Autodesk Inventor part; units mm, degrees
ref_plane "YZ Plane" through (0, 0, 0) normal (1, 0, 0) x (0, 1, 0)
ref_plane "XZ Plane" through (0, 0, 0) normal (0, 1, 0) x (-1, 0, 0)
ref_plane "XY Plane" through (0, 0, 0) normal (0, 0, 1) x (1, 0, 0)
sketch "Sketch1" plane through (0, 0, 0) normal (0, 0, 1) x (1, 0, 0)
  line L0 (14, -20) -> (-14, -20) construction
  line L1 (-14, -20) -> (-14, 20) construction
  line L2 (-14, 20) -> (14, 20) construction
  line L3 (14, 20) -> (14, -20) construction
  line L4 (14, -20) -> (-14, 20) construction
  line L5 (-14, -20) -> (14, 20) construction
  circle A0 centre (-14, 20) radius 2.25
  circle A1 centre (14, 20) radius 2.25
  circle A2 centre (14, -20) radius 2.25
  circle A3 centre (-14, -20) radius 2.25
  line L6 (0, 0) -> (0, -8.85) construction
  circle A4 centre (0, -8.85) radius 10
  line L7 (20.06, -29.05) -> (-20.06, -29.05)
  line L8 (-20.06, -29.05) -> (-20.06, 29.05)
  line L9 (-20.06, 29.05) -> (20.06, 29.05)
  line L10 (20.06, 29.05) -> (20.06, -29.05)
  line L11 (20.06, -29.05) -> (-20.06, 29.05) construction
  line L12 (-20.06, -29.05) -> (20.06, 29.05) construction
  dimension "d0" = 28
  dimension "d1" = 40
  dimension "d2" = 20
  dimension "d3" = 4.5
  dimension "d4" = 58.1
  dimension "d5" = 40.12
  dimension "d6" = 37.9
extrude "Extrusion1" add sketch "Sketch1" along normal blind 8
sketch "Sketch2" plane through (0, 0, 8) normal (0, 0, 1) x (1, 0, 0)
  circle A0 centre (0, -8.85) radius 10 construction
  circle A1 centre (-14, -20) radius 2.25 construction
  circle A2 centre (14, -20) radius 2.25 construction
  circle A3 centre (14, 20) radius 2.25 construction
  circle A4 centre (-14, 20) radius 2.25 construction
  line L0 (-20.06, -29.05) -> (20.06, -29.05) construction
  line L1 (20.06, -29.05) -> (20.06, 29.05) construction
  line L2 (20.06, 29.05) -> (-20.06, 29.05) construction
  line L3 (-20.06, 29.05) -> (-20.06, -29.05) construction
  circle A5 centre (14, -20) radius 3.5
  circle A6 centre (-14, -20) radius 3.5
  circle A7 centre (14, 20) radius 3.5
  circle A8 centre (-14, 20) radius 3.5
  point P0 (0, 0)
  dimension "d9" = 7
extrude "Extrusion2" cut sketch "Sketch2" against normal blind 4
sketch "Sketch3" plane through (-20.06, 29.05, 0) normal (0, 1, 0) x (1, 0, 0)
  line L0 (40.12, 0) -> (0, 0)
  line L1 (0, 0) -> (0, -12)
  line L2 (0, -12) -> (40.12, -12)
  line L3 (40.12, -12) -> (40.12, 0)
  circle A0 centre (20.06, 19.7) radius 15.5 construction
  line L4 (40.12, 0) -> (33.3508, 11.7247)
  line L5 (0, 0) -> (6.7692, 11.7247)
  arc A1 (6.7692, 11.7247) -> (33.3508, 11.7247) centre (20.06, 19.7) ccw
  line L6 (40.12, 0) -> (0, 0)
  line L7 (40.12, 0) -> (0, 0)
  point P0 (20.06, 0)
  dimension "d12" = 12
  dimension "d19" = 60
extrude "Extrusion3" add sketch "Sketch3" along normal blind 40
sketch "Sketch4" plane through (-20.06, 69.05, 0) normal (0, 1, 0) x (1, 0, 0)
  line L0 (20.06, 0) -> (20.06, -27) construction
  circle A0 centre (20.06, -27) radius 8
  line L1 (20.06, -27) -> (20.06, 0) construction
  line L2 (40.12, 0) -> (0, 0)
  line L3 (40.12, -27) -> (40.12, 0)
  line L4 (0, 0) -> (0, -27)
  arc A1 (0, -27) -> (40.12, -27) centre (20.06, -27) ccw
  arc A2 (40.12, 0) -> (0, 0) centre (20.06, 0) ccw construction
  line L5 (40.12, 0) -> (40.12, -8)
  line L6 (40.12, 0) -> (0, 0)
  line L7 (0, 0) -> (40.12, 0)
  line L8 (40.12, 0) -> (33.3508, 11.7247)
  arc A3 (6.7692, 11.7247) -> (33.3508, 11.7247) centre (20.06, 19.7) ccw
  line L9 (6.7692, 11.7247) -> (0, 0)
  line L10 (0, 0) -> (0, -12)
  line L11 (0, -12) -> (40.12, -12)
  line L12 (40.12, -12) -> (40.12, 0)
  point P0 (20.06, -13.5)
  dimension "d15" = 27
  dimension "d16" = 16
extrude "Extrusion4" add sketch "Sketch4" along normal blind 6
sketch "Sketch5" plane through (-20.06, -29.05, 0) normal (0, -1, 0) x (1, 0, 0)
  line L0 (40.12, 0) -> (40.12, 8)
  line L1 (40.12, 8) -> (65.12, 8)
  line L2 (65.12, 8) -> (65.12, -17)
  line L3 (65.12, -17) -> (40.12, -17)
  line L4 (40.12, -17) -> (40.12, 8)
  line L5 (40.12, 0) -> (33.3508, -11.7247)
  line L6 (33.3508, -11.7247) -> (40.12, -17)
  line L7 (40.12, 27) -> (40.12, 0)
  line L8 (40.12, -17) -> (40.12, 0)
  point P0 (20.06, 0)
  dimension "d20" = 25
  dimension "d21" = 25
extrude "Extrusion5" add sketch "Sketch5" against normal up to surface (58.1 mm away) contours L0 L1 L2 L3 L4
sketch "Sketch6" plane through (20.06, 29.05, -17) normal (0, 1, 0) x (1, 0, 0)
  line L0 (25, 0) -> (0, 0)
  line L1 (0, 0) -> (0, -17)
  line L2 (0, -25) -> (0, -17)
  line L3 (0, -25) -> (25, -25)
  line L4 (25, -25) -> (25, 0)
  line L5 (0, -17) -> (-6.7692, -5.2753)
  line L6 (25, 0) -> (0, 0)
  line L7 (0, 0) -> (-6.7692, -5.2753)
  line L8 (0, 0) -> (0, -17)
  line L9 (0, -17) -> (0, 0)
  point P0 (-20.06, -17)
extrude "Extrusion6" add sketch "Sketch6" along normal up to surface (46 mm away)
sketch "Sketch7" plane through (45.06, -29.05, 8) normal (1, 0, 0) x (0, 0, -1)
  line L0 (25, 104.1) -> (0, 104.1)
  line L1 (25, 0) -> (25, 104.1)
  line L2 (25, 104.1) -> (25, 0)
  line L3 (25, 0) -> (45, 0)
  line L4 (45, 0) -> (45, 104.1)
  line L5 (45, 104.1) -> (25, 104.1)
  point P0 (8, 29.05)
  dimension "d26" = 20
extrude "Extrusion7" add sketch "Sketch7" against normal blind 10
sketch "Sketch8" plane through (35.06, -29.05, 8) normal (-1, 0, 0) x (0, 0, 1)
  line L0 (-25, 104.1) -> (-25, 0)
  line L1 (-25, 104.1) -> (-45, 104.1)
  line L2 (-45, 104.1) -> (-45, 0)
  line L3 (-45, 0) -> (-25, 0)
  line L4 (-45, 104.1) -> (-45, 0)
  line L5 (-45, 52.05) -> (-25, 52.05) construction
  line L6 (-35, 84.55) -> (-35, 19.55) construction
  circle A0 centre (-35, 84.55) radius 2.5
  circle A1 centre (-35, 19.55) radius 2.5
  point P0 (-8, 29.05)
  point P1 (-35, 52.05)
  dimension "d29" = 65
  dimension "d30" = 5
extrude "Extrusion8" cut sketch "Sketch8" against normal through all contours A0 | A1
chamfer "Chamfer1" distance 4 angle 45 5 edges at (40.06, 75.05, -37) (40.06, -29.05, -37) (27.56, -29.05, -17) (-20.06, -29.05, 4) (0, 29.05, 12)
sketch "Sketch9" plane through (-20.06, 75.05, 0) normal (0, 1, 0) x (1, 0, 0)
  circle A0 centre (20.06, 19.7) radius 15.5 construction
  circle A1 centre (20.06, 19.7) radius 16.5
  point P0 (20.06, 0)
  dimension "d36" = 1
extrude "Extrusion9" cut sketch "Sketch9" against normal up to surface (46 mm away)
properties part number "frame"
Geometry: final body of the model. Coordinates: model frame, mm. A direction names the side the tool comes from. Give positions to 0.01 mm unless a question says otherwise; leave off trailing zeros. Write each loop counter-clockwise with the first axis right and the second up, starting at its lowest first coordinate (ties: lowest second). Pieces come first, ordered by that corner, then holes. Notation, with made-up numbers: (33, 68) -> (65, 68) arc R21 cw to (65, 97) -> close; hole circle Ø7 at (21, -16.5). An arc over 180 degrees is marked (long way). Answer as a JSON object with one key per item and string values.
1. Cut plane C-C on z = 30.5. Output: boundary loops of the cut face in (x, y).
Ans:
{"outline": "(-19.75, 69.05) -> (-7.19, 69.05) -> (-7.19, 75.05) -> (-19.75, 75.05) -> close; (7.19, 69.05) -> (19.75, 69.05) -> (19.75, 75.05) -> (7.19, 75.05) -> close"}
2. Cut plane B-B on y = 55.5. Output: boundary loops of the cut face in (x, z), and give its area (3 significant figures).
Ans:
{"outline": "(-20.06, 0) -> (-13.86, -10.74) arc R16.5 cw to (15.16, -13.18) -> (20.06, -17) -> (35.06, -17) -> (35.06, -24.5) -> (45.06, -24.5) -> (45.06, 8) -> (20.06, 8) -> (20.06, 12) -> (-20.06, 12) -> close; (35.06, -37) -> (45.06, -37) -> (45.06, -29.5) -> (35.06, -29.5) -> close", "area": "1,530 mm^2"}
3. Contact query for flat-ended pins moving along their axis: pin 1 (7.5 mm diameter, centred on x = 14, y = -20, fed in from +Z); pin 2 (1 mm diameter, centred on x = 1.5, y = 52.5, fed in from -Z); pin 3 (1 mm diameter, centred on x = 33, y = -1.5, fed in from -Z); pin 4 (4 mm diameter, centred on x = 14, y = -20, fed in from -Z). Output: stop coordinate, or through.
Ans:
{"pin 1": "stops at z = 8", "pin 2": "stops at z = -3.32", "pin 3": "stops at z = -17", "pin 4": "passes through"}
4. Ray query, probe 1 along Y at (x, z) = (14, 6); probe 2 along X at (y, z) = (20, 2.8); probe 3 along Y at (x, z) = (40.75, -27). Return the intervals inside material, ascending. Write a range as from..to.
Ans:
{"probe 1": "y = -29.05..-23.5, -16.5..16.5, 23.5..75.05", "probe 2": "x = -20.06..-16.25, -11.75..11.75, 16.25..45.06", "probe 3": "y = -29.05..-12, -7..53, 58..75.05"}
5. Cut plane D-D on y = 20. Output: boundary loops of the cut face in (x, z).
Ans:
{"outline": "(-20.06, 0) -> (-16.25, 0) -> (-16.25, 4) -> (-17.5, 4) -> (-17.5, 8) -> (-20.06, 8) -> close; (-11.75, 0) -> (11.75, 0) -> (11.75, 4) -> (10.5, 4) -> (10.5, 8) -> (-10.5, 8) -> (-10.5, 4) -> (-11.75, 4) -> close; (16.25, 0) -> (20.06, 0) -> (20.06, -17) -> (35.06, -17) -> (35.06, -37) -> (45.06, -37) -> (45.06, 8) -> (17.5, 8) -> (17.5, 4) -> (16.25, 4) -> close"}
6. Cut plane A-A on x = 0. Count the separate pieces of the cut face and the enclosed holes in it, and give its area (3 significant figures).
Ans:
{"separate pieces": "3", "enclosed holes": "0", "area": "1,110 mm^2"}
7. Access query for faces 1 (the cylindrical face through (13.54, -16.53, 6.03)), 2 (the cylindrical face through (13.512, 22.196, 1.972)), 3 (the flat face through (19, 11, 8)), 4 (the flat face through (9, 69.05, 29)), 5 (the flat face through (4, 29.05, -3)). Directions: +Z, -Z, +X, -X, +Y, -Y. A direction counts if a zero-diameter tool reaches every point of the face in a straight line with its end or side. Return the directions, or none.
Ans:
{"face 1": "+Z", "face 2": "+Z, -Z", "face 3": "+Z, +X, -Y", "face 4": "+Z, +X, -X, -Y", "face 5": "-Z, -X, -Y"}
8. Mould query, pull axis X, two halves, no side actions, for faces 6 (the flat face through (20.06, 59, 11)), 7 (the flat face through (0, 51, 12)), 8 (the cylindrical face through (-12.12, 22.95, 6.03)). Classes: pulls with the +X half, pulls with the -X half, needs draft (parallel to the pull), parting line crosses it, or undercut.
Ans:
{"face 6": "pulls with the +X half", "face 7": "needs draft", "face 8": "undercut"}
